Design review of the part built by this model. Coordinates are the model's own, in mm. Face numbers are marked on the shaded views. A direction names the side the tool comes from. Coordinates: 2 decimals unless noted, no trailing zeros. Loops run counter-clockwise (first coordinate to the right, second up) from the corner with the lowest first, then second, coordinate; pieces in that order, holes last. Notation, with made-up numbers: (-9, -36) -> (16, -36) arc R10 ccw to (16, -30) -> close; hole circle Ø3 at (6, 69.5). An arc over 180 degrees is marked (long way). Answer in a Markdown table with one row per item.
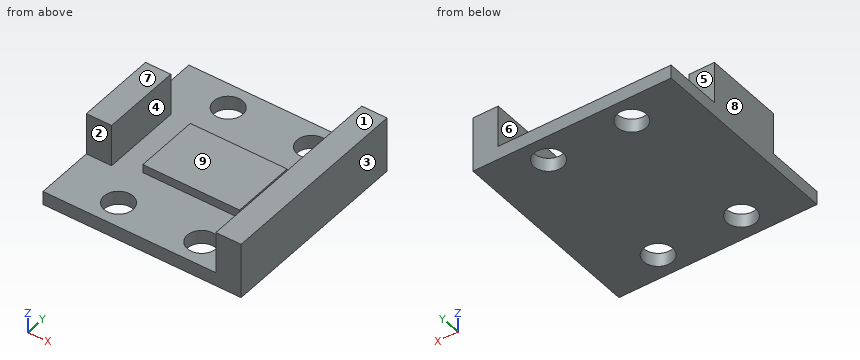
```python
from build123d import *

# Parameters (mm, degrees)
F0_W     = 23.55
F0_H     = 23.55
F0_R     = 1.725
F1_DEPTH = 1.62
F2_W     = 3
F2_H     = 23.55
F2_H_2   = 9.55
F3_DEPTH = 5
F4_W     = 11.512548
F4_H     = 7.665078
F5_DEPTH = 1


with BuildPart() as f1:
    # F0 (on Top) → F1 (new body)
    with BuildSketch(Plane.XY):
        Rectangle(F0_W, F0_H)
        with Locations((-4.95, -8.85)):
            Circle(F0_R, mode=Mode.SUBTRACT)
        with Locations((4.95, -8.85)):
            Circle(F0_R, mode=Mode.SUBTRACT)
        with Locations((-4.95, 8.85)):
            Circle(F0_R, mode=Mode.SUBTRACT)
        with Locations((4.95, 8.85)):
            Circle(F0_R, mode=Mode.SUBTRACT)
    extrude(amount=F1_DEPTH)

    # F2 (on face) → F3 (join)
    with BuildSketch(Plane.XY.offset(1.62)):
        with Locations((10.275, 0)):
            Rectangle(F2_W, F2_H)
        with Locations((-10.275, 0)):
            Rectangle(F2_W, F2_H_2)
    extrude(amount=F3_DEPTH)

    # F4 (on face) → F5 (join)
    with BuildSketch(Plane.XY.offset(1.62)):
        Rectangle(F4_W, F4_H)
    extrude(amount=F5_DEPTH)


solid = f1.part
```
(1) Take a section at D-D on z = 1. Give the boundary of the cut face in (x, y) (3 decimals), and give its area (3 significant figures).
Evaluation:
| item | result |
|---|---|
| outline | (-11.775, -11.775) -> (11.775, -11.775) -> (11.775, 11.775) -> (-11.775, 11.775) -> close; hole circle Ø3.45 at (-4.95, -8.85); hole circle Ø3.45 at (-4.95, 8.85); hole circle Ø3.45 at (4.95, -8.85); hole circle Ø3.45 at (4.95, 8.85) |
| area | 517 mm² |
(2) Take a section at B-B on z = 3.5. Give the boundary of the cut face in (x, y) (3 decimals), and give its area (3 significant figures).
Evaluation:
| item | result |
|---|---|
| outline | (-11.775, -4.775) -> (-8.775, -4.775) -> (-8.775, 4.775) -> (-11.775, 4.775) -> close; (8.775, -11.775) -> (11.775, -11.775) -> (11.775, 11.775) -> (8.775, 11.775) -> close |
| area | 99.3 mm² |
(3) Draft analysis for pull direction X (two halves, no side actions). For the marked faces 6, 7, 8 and 9, state which applies: pulls with the +X half, pulls with the -X half, needs draft (parallel to the pull), parting line crosses it, or undercut.
Evaluation:
| item | result |
|---|---|
| face 6 | undercut |
| face 7 | needs draft |
| face 8 | pulls with the -X half |
| face 9 | undercut |
(4) For pin 1 (1 mm diameter, centred on x = -3, y = 1.5, fed in from +Z); pin 2 (1.5 mm diameter, centred on x = -9.5, z = 5.5, fed in from +Y) (3 decimals); pin 3 (0.5 mm diameter, centred on x = -1, z = 2.5, fed in from +Y); pin 4 (3 mm diameter, centred on x = 4.95, y = -8.85, fed in from -Z), all flat-tipped, find the tip position at first contact; note any pin that passes through.
Evaluation:
| item | result |
|---|---|
| pin 1 | stops at z = 2.62 |
| pin 2 | stops at y = 4.775 |
| pin 3 | stops at y = 3.83 |
| pin 4 | passes through |
(5) To check wall thickness, follow probe 1 along Y at (x, z) = (-4.95, 1.2) (3 decimals); probe 2 along X at (y, z) = (-2.25, 3.5) (3 decimals); probe 3 along Z at (x, y) = (-10, -5). State the ranges of each line that lie inside material, in increasing order.
Evaluation:
| item | result |
|---|---|
| probe 1 | y = -11.775 to -10.575, -7.125 to 7.125, 10.575 to 11.775 |
| probe 2 | x = -11.775 to -8.775, 8.775 to 11.775 |
| probe 3 | z = 0 to 1.62 |
(6) Take a section at A-A on x = -4.95. Give the boundary of the cut face in (y, z) (3 decimals), and give its area (3 significant figures).
Evaluation:
| item | result |
|---|---|
| outline | (-11.775, 0) -> (-10.575, 0) -> (-10.575, 1.62) -> (-11.775, 1.62) -> close; (-7.125, 0) -> (7.125, 0) -> (7.125, 1.62) -> (3.833, 1.62) -> (3.833, 2.62) -> (-3.833, 2.62) -> (-3.833, 1.62) -> (-7.125, 1.62) -> close; (10.575, 0) -> (11.775, 0) -> (11.775, 1.62) -> (10.575, 1.62) -> close |
| area | 34.6 mm² |
(7) Tool access review of the marked faces 1, 2, 3, 4 and 5: name each direction out of +Z, -Z, +X, -X, +Y, -Y from which nothing blocks a thin tool from reaching the whole face with its end or side.
Evaluation:
| item | result |
|---|---|
| face 1 | +Z, +X, -X, +Y, -Y |
| face 2 | +Z, -X, -Y |
| face 3 | +Z, -Z, +X, +Y, -Y |
| face 4 | +Z, +Y, -Y |
| face 5 | +Z, -X, +Y |
(8) Take a section at C-C on y = -8.85. Give the boundary of the cut face in (x, z) (3 decimals).
Evaluation:
| item | result |
|---|---|
| outline | (-11.775, 0) -> (-6.675, 0) -> (-6.675, 1.62) -> (-11.775, 1.62) -> close; (-3.225, 0) -> (3.225, 0) -> (3.225, 1.62) -> (-3.225, 1.62) -> close; (6.675, 0) -> (11.775, 0) -> (11.775, 6.62) -> (8.775, 6.62) -> (8.775, 1.62) -> (6.675, 1.62) -> close |
